Could you check a few things on this model? Use its own coordinates, in mm. A direction names the side the tool comes from. Coordinates: 2 decimals unless noted, no trailing zeros. Loops run counter-clockwise (first coordinate to the right, second up) from the corner with the lowest first, then second, coordinate; pieces in that order, holes last. Notation, with made-up numbers: M 34,10 L 88,10 A16 ccw 88,30 Z; hole C 25.25,83 d11. An arc over 180 degrees is marked long. Write each question's results on one line, items separated by ' | '.
```python
from build123d import *

# Parameters (mm, degrees)
SKETCH1_R           = 17.4625
SKETCH1_R_2         = 2.4257
SKETCH1_R_3         = 7.9375
BOSS_EXTRUDE1_DEPTH = 3.175


with BuildPart() as part:
    # Sketch1 → Boss-Extrude1 (new body)
    with BuildSketch(Plane(origin=(0, 0, 0), x_dir=(1, 0, 0), z_dir=(0, 1, 0))):
        Polygon((0, 0), (876.3, 0), (876.3, 165.1), (698.5, 165.1), (609.6, 76.2), (127, 76.2), (38.1, 165.1), (0, 165.1), align=None)
        with Locations(Location((214.9475, 38.9255, 0), (0, 0, 270))):
            Circle(SKETCH1_R, mode=Mode.SUBTRACT)
        with Locations(Location((712.16774, 87.9475, 0), (0, 0, 270))):
            Circle(SKETCH1_R, mode=Mode.SUBTRACT)
        with Locations(Location((438.15, 15.875, 0), (0, 0, 270))):
            Circle(SKETCH1_R_2, mode=Mode.SUBTRACT)
        with Locations(Location((539.75, 15.875, 0), (0, 0, 270))):
            Circle(SKETCH1_R_2, mode=Mode.SUBTRACT)
        with Locations(Location((641.35, 15.875, 0), (0, 0, 270))):
            Circle(SKETCH1_R_2, mode=Mode.SUBTRACT)
        with Locations(Location((742.95, 15.875, 0), (0, 0, 270))):
            Circle(SKETCH1_R_2, mode=Mode.SUBTRACT)
        with Locations(Location((844.55, 15.875, 0), (0, 0, 270))):
            Circle(SKETCH1_R_2, mode=Mode.SUBTRACT)
        with Locations(Location((31.75, 15.875, 0), (0, 0, 270))):
            Circle(SKETCH1_R_2, mode=Mode.SUBTRACT)
        with Locations(Location((133.35, 15.875, 0), (0, 0, 270))):
            Circle(SKETCH1_R_2, mode=Mode.SUBTRACT)
        with Locations(Location((234.95, 15.875, 0), (0, 0, 270))):
            Circle(SKETCH1_R_2, mode=Mode.SUBTRACT)
        with Locations(Location((336.55, 15.875, 0), (0, 0, 270))):
            Circle(SKETCH1_R_2, mode=Mode.SUBTRACT)
        with Locations(Location((16.637, 53.975, 0), (0, 0, 270))):
            Circle(SKETCH1_R_2, mode=Mode.SUBTRACT)
        with Locations(Location((16.637, 79.375, 0), (0, 0, 270))):
            Circle(SKETCH1_R_2, mode=Mode.SUBTRACT)
        with Locations(Location((16.637, 104.775, 0), (0, 0, 270))):
            Circle(SKETCH1_R_2, mode=Mode.SUBTRACT)
        with Locations(Location((16.637, 130.175, 0), (0, 0, 270))):
            Circle(SKETCH1_R_2, mode=Mode.SUBTRACT)
        with Locations(Location((859.663, 53.975, 0), (0, 0, 270))):
            Circle(SKETCH1_R_2, mode=Mode.SUBTRACT)
        with Locations(Location((859.663, 79.375, 0), (0, 0, 270))):
            Circle(SKETCH1_R_2, mode=Mode.SUBTRACT)
        with Locations(Location((859.663, 104.775, 0), (0, 0, 270))):
            Circle(SKETCH1_R_2, mode=Mode.SUBTRACT)
        with Locations(Location((859.663, 130.175, 0), (0, 0, 270))):
            Circle(SKETCH1_R_2, mode=Mode.SUBTRACT)
        with Locations(Location((82.55, 15.875, 0), (0, 0, 270))):
            Circle(SKETCH1_R_2, mode=Mode.SUBTRACT)
        with Locations(Location((793.75, 15.875, 0), (0, 0, 270))):
            Circle(SKETCH1_R_2, mode=Mode.SUBTRACT)
        with Locations(Location((19.05, 149.225, 0), (0, 0, 270))):
            Circle(SKETCH1_R_3, mode=Mode.SUBTRACT)
    extrude(amount=BOSS_EXTRUDE1_DEPTH)


solid = part.part
```
(1) Which directions (+Z, -Z, +X, -X, +Y, -Y) give clear straight access to the entire face, cutting with the end or side of a thin tool? Please do faces 4 (the flat face through (432, 3.175, -65)), 5 (the flat face through (83.2, 1.6, -120)).
Reported:
face 4: +Z, -Z, +X, -X, +Y | face 5: -Z, +Y, -Y
(2) Imagine slicing it at A-A, the plane y = 2.35. State how many separate pieces and enclosed holes the cut face has, and give its area (3 significant figures).
Reported:
separate pieces: 1 | enclosed holes: 22 | area: 91,400 mm2
(3) Please list where these lines run through material, in increasing order: probe 1 along X at (y, z) = (2.1, -129.5); probe 2 along X at (y, z) = (2.15, -38); probe 3 along Z at (x, y) = (234.95, 2). Write a range as from..to.
Reported:
probe 1: x = 0..14.31, 18.97..73.7, 662.9..857.33, 861.99..876.3 | probe 2: x = 0..197.51, 232.39..876.3 | probe 3: z = -76.2..-18.3, -13.45..0
(4) Imagine slicing it at B-B, the plane x = 246. List the corners of the cut face in (y, z) for me (3 decimals).
Reported:
outline: M 0,-76.2 L 3.175,-76.2 L 3.175,0 L 0,0 Z
(5) If we mould it in two halves opening along X, with no side actions, what happens to faces 1 (the flat face through (654.7, 1.6, -121.3)), 2 (the flat face through (432, 0, -65)), 3 (the cylindrical face through (229.672, 1.565, -29.538))? For each: released by +X, released by -X, zero draft, split by the parting line, or undercut.
Reported:
face 1: undercut | face 2: zero draft | face 3: undercut
(6) Will this pin go through, and if not, where does the flat tip stop? P1, Ø3, axis at x = 859.663, z = -79.375, coming from the -Y side.
Reported:
P1: passes through
